Design review of the part built by this model. Coordinates are the model's own, in mm. A direction names the side the tool comes from. Give positions to 0.01 mm unless a question says otherwise; leave off trailing zeros. Loops run counter-clockwise (first coordinate to the right, second up) from the corner with the lowest first, then second, coordinate; pieces in that order, holes last.
from build123d import *

# Parameters (mm, degrees)
REVOLUTION_ANGLE = 90
POCKET_DEPTH     = 10.001
FILLET_R         = 1


with BuildPart() as part:
    # Sketch001 → Revolution (revolve)
    with BuildSketch(Plane.XZ):
        with BuildLine():
            ThreePointArc((19.93934, 8), (18.842964, 9.44949), (17.110913, 10))
            Line((17.110913, 8), (17.110913, 10))
            Line((16.110913, 8), (17.110913, 8))
            Line((16.110913, 3), (16.110913, 8))
            Line((17.5, 3), (16.110913, 3))
            Line((17.5, 0), (17.5, 3))
            Line((18.5, 0), (17.5, 0))
            Line((20, 2), (18.5, 0))
            Line((20, 2), (21, 2))
            Line((21, 2), (28.65, 0))
            Line((28.65, 1.5), (28.65, 0))
            Line((21, 5), (28.65, 1.5))
            Line((19.93934, 8), (21, 5))
        make_face()
    revolve(axis=Axis((0, 0, 0), (0, 0, 1)), revolution_arc=REVOLUTION_ANGLE)

    # Sketch002 → Pocket (cut, through all)
    with BuildSketch(Plane.XY):
        with BuildLine():
            Line((10, 17.320508), (10, 25))
            Line((10, 25), (14, 25))
            Line((14, 25), (14, 14.282857))
            ThreePointArc((20, 0), (18.439089, 7.745967), (14, 14.282857))
            Line((37.402618, 0), (20, 0))
            Line((37.402618, 41.95618), (37.402618, 0))
            Line((0, 41.95618), (37.402618, 41.95618))
            Line((0, 20), (0, 41.95618))
            ThreePointArc((10, 17.320508), (5.176381, 19.318517), (0, 20))
        make_face()
    extrude(amount=POCKET_DEPTH, mode=Mode.SUBTRACT)

    # Fillet
    fillet_edges = [part.edges().sort_by_distance(p)[0] for p in [
        (12.001906, 25, 1.920149),
    ]]
    fillet(fillet_edges, radius=FILLET_R)


solid = part.part
Q1. Insertion check: pin 1 (2 mm diameter, centred on y = 11, z = 5, fed in from +X); pin 2 (5 mm diameter, centred on x = 12.5, y = 10, fed in from -Z); pin 3 (5 mm diameter, centred on x = 6.5, y = 20.5, fed in from -Z); pin 4 (4 mm diameter, centred on y = 19.5, z = 5.5, fed in from +X). Each pin has a flat end and moves straight along its axis. Give the tip position at first contact, or say it passes through.
Results:
pin 1: stops at x = 17.32
pin 2: stops at z = 0
pin 3: stops at z = 0.67
pin 4: stops at x = 14
Q2. Take a section at A-A (z = 5.75). Give the boundary of the cut face in (x, y), plus the area to 3 significant figures.
Results:
outline: (0, 16.11) arc R16.11 cw to (16.11, 0) - (20, 0) arc R20 ccw to (14, 14.28) - (14, 15.29) arc R20.73 ccw to (10, 18.16) - (10, 17.32) arc R20 ccw to (0, 20) - close
area: 114 mm2
Q3. Take a section at C-C (z = 8.75). Give the boundary of the cut face in (x, y), plus the area to 3 significant figures.
Results:
outline: (0, 17.11) arc R17.11 cw to (17.11, 0) - (19.55, 0) arc R19.55 ccw to (0, 19.55) - close
area: 70.2 mm2
Q4. Wall thickness on line 1 (Z direction, x = 9.75, y = 14); line 2 (Z direction, x = 17, y = 2.75); line 3 (X direction, y = 18, z = 5.75): over which ranges is each line inside the solid? List them lowest first.
Results:
line 1: z = 3 to 8
line 2: z = 3 to 10
line 3: x = 0 to 8.72, 10 to 10.29
Q5. Tool access review of faces 1 (the face through (11, 12, 8)), 2 (the face through (12.51, 12.24, 1.52)), 3 (the face through (11.91, 20.87, 1.21)): name each direction out of +Z, -Z, +X, -X, +Y, -Y from which nothing blocks a thin tool from reaching the whole face with its end or side.
Results:
face 1: +Z, -X, -Y
face 2: -Z, -X, -Y
face 3: -Z
Q6. Draft analysis for pull direction Y (two halves, no side actions). For faces 4 (the face through (12, 16.4, 2)), 5 (the face through (12.2, 12, 9)), 6 (the face through (14, 19, 2)), 7 (the face through (18.5, 7.6, 4.9)), state which applies: pulls with the +Y half, pulls with the -Y half, needs draft (parallel to the pull), parting line crosses it, or undercut.
Results:
face 4: undercut
face 5: pulls with the -Y half
face 6: needs draft
face 7: pulls with the +Y half
Q7. Take a section at B-B (z = 7.25). Give the boundary of the cut face in (x, y).
Results:
outline: (0, 16.11) arc R16.11 cw to (16.11, 0) - (20, 0) arc R20 ccw to (14, 14.28) - (14, 14.57) arc R20.2 ccw to (10, 17.56) - (10, 17.32) arc R20 ccw to (0, 20) - close
